Here's the drawing with two shaded views (mm, measured from the low corner). I have some questions. Coordinates: 2 decimals unless noted, no trailing zeros. Write each loop counter-clockwise with the first axis right and the second up, starting at its lowest first coordinate (ties: lowest second). Pieces come first, ordered by that corner, then holes.
Item 1: If I drill on probe 1 along Y at (x, z) = (6, 2); probe 2 along Y at (x, z) = (4.75, 8); probe 3 along X at (y, z) = (5.5, 7), over which ranges is the centre line in solid material (lowest first)?
Item 2: I want a section at C-C on z = 4.25. Please give me the cut outline in (x, y), then the cut area to 3 significant figures.
Item 3: I want a section at A-A on x = 6. Please give me the cut outline in (y, z), then the cut area to 3 significant figures.
Item 4: For P1, Ø2, axis at x = 2, z = 3, coming from the +Y side; P2, Ø4, axis at x = 4, z = 9, coming from the -Y side; P3, Ø2, axis at y = 3, z = 7, coming from the +X side, each with a flat end and sliding along its axis, tell me the tip position at first contact or that it passes through.
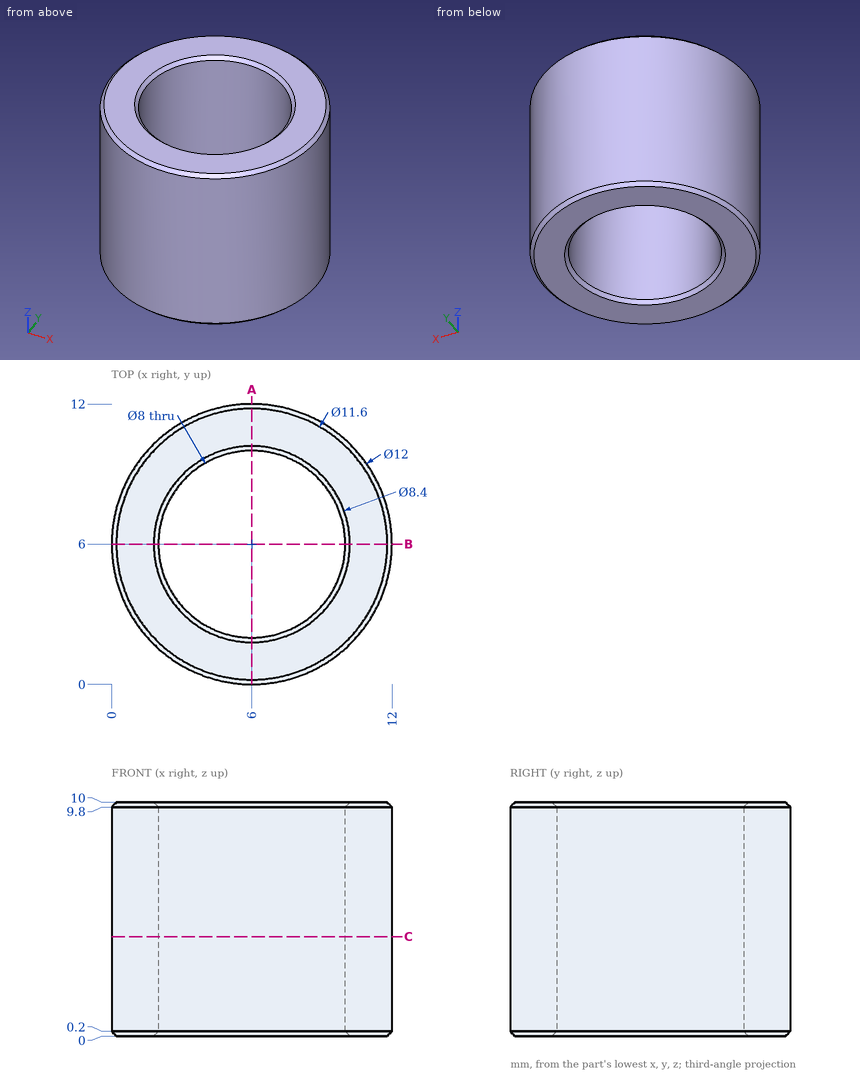
Response values:
1. probe 1: y = 0 to 2, 10 to 12
1. probe 2: y = 0.13 to 2.2, 9.8 to 11.87
1. probe 3: x = 0.02 to 2.03, 9.97 to 11.98
2. outline: circle Ø12 at (6, 6); hole circle Ø8 at (6, 6)
2. area: 62.8 mm2
3. outline: (0, 0.2) - (0.2, 0) - (1.8, 0) - (2, 0.2) - (2, 9.8) - (1.8, 10) - (0.2, 10) - (0, 9.8) - close; (10, 0.2) - (10.2, 0) - (11.8, 0) - (12, 0.2) - (12, 9.8) - (11.8, 10) - (10.2, 10) - (10, 9.8) - close
3. area: 39.8 mm2
4. P1: stops at y = 11.2
4. P2: stops at y = 0
4. P3: stops at x = 11.66
